Autodesk Inventor part; units mm, degrees
ref_plane "YZ Plane" through (0, 0, 0) normal (1, 0, 0) x (0, 1, 0)
ref_plane "XZ Plane" through (0, 0, 0) normal (0, 1, 0) x (-1, 0, 0)
ref_plane "XY Plane" through (0, 0, 0) normal (0, 0, 1) x (1, 0, 0)
sketch "Sketch1" plane through (0, 0, 0) normal (1, 0, 0) x (0, 1, 0)
  line L0 (0, 0) -> (20, 0)
  line L1 (20, 0) -> (20, -160)
  line L2 (20, -160) -> (0, -160)
  line L3 (0, -160) -> (0, 0)
  line L4 (10, 0) -> (10, -160) construction
  line L5 (20, -6) -> (0, -6) construction
  line L6 (20, -16) -> (0, -16) construction
  line L7 (20, -142.5) -> (0, -142.5) construction
  line L8 (25, -152.5) -> (0, -152.5) construction
  line L9 (20, -89) -> (0, -89) construction
  line L10 (25, -99) -> (0, -99) construction
  point P0 (15, -16)
  point P1 (15, -6)
  point P2 (5, -16)
  point P3 (5, -6)
  point P4 (15, -152.5)
  point P5 (15, -142.5)
  point P6 (5, -142.5)
  point P7 (5, -152.5)
  point P8 (15, -99)
  point P9 (15, -89)
  point P10 (5, -89)
  point P11 (5, -99)
  dimension "d1" = 20
  dimension "d10" = 6
  dimension "d11" = 10
  dimension "d12" = 10
  dimension "d13" = 10
  dimension "d14" = 10
  dimension "d16" = 10
  dimension "d17" = 10
  dimension "d27" = 10
  dimension "d28" = 10
  dimension "d29" = 10
  dimension "d30" = 89
  dimension "d40" = 142.5
  dimension "d41" = 160
extrude "Extrusion1" add sketch "Sketch1" along normal blind 2
hole "Hole1" at (0, 15, -16) at (0, 15, -6) at (0, 5, -16) at (0, 5, -6) at (0, 15, -142.5) at (0, 15, -152.5) at (0, 5, -152.5) at (0, 5, -142.5) at (0, 15, -89) at (0, 15, -99) at (0, 5, -99) at (0, 5, -89) direction (1, 0, 0) diameter 5 end through all
sketch "Sketch2" plane through (2, 0, 0) normal (1, 0, 0) x (0, 0, -1)
  arc A0 (27.5, 16) -> (27.5, 4) centre (27.5, 10) ccw
  line L0 (27.5, 10) -> (27.5, 4) construction
  line L1 (27.5, 10) -> (27.5, 16) construction
  line L2 (0, 20) -> (0, 0)
  line L3 (0, 10) -> (160, 10) construction
  line L4 (160, 0) -> (160, 20)
  line L5 (27.5, 16) -> (77.5, 16)
  line L6 (27.5, 4) -> (77.5, 4)
  circle A1 centre (89, 15) radius 2.5 construction
  circle A2 centre (89, 5) radius 2.5 construction
  line L7 (89, 15) -> (89, 5) construction
  circle A3 centre (16, 15) radius 2.5 construction
  circle A4 centre (16, 5) radius 2.5 construction
  line L8 (16, 15) -> (16, 5) construction
  circle A5 centre (99, 15) radius 2.5 construction
  line L9 (99, 15) -> (89, 15) construction
  line L10 (94, 15) -> (94, -7.3428) construction
  arc A6 (77.5, 4) -> (77.5, 16) centre (77.5, 10) ccw
  line L11 (77.5, 10) -> (77.5, 4) construction
  line L12 (77.5, 10) -> (77.5, 16) construction
  line L13 (110.5, 4) -> (131, 4)
  line L14 (131, 16) -> (110.5, 16)
  arc A7 (110.5, 16) -> (110.5, 4) centre (110.5, 10) ccw
  arc A8 (131, 4) -> (131, 16) centre (131, 10) ccw
  circle A9 centre (99, 5) radius 2.5 construction
  circle A10 centre (16, 15) radius 2.5 construction
  circle A11 centre (142.5, 5) radius 2.5 construction
  dimension "d31" = 180
  dimension "d32" = 6
  dimension "d33" = 50
  dimension "d34" = 73
  dimension "d36" = 180
  dimension "d42" = 6
  dimension "d43" = 6
  dimension "d44" = 20.5
  dimension "d46" = 180
  dimension "d47" = 5
  dimension "d48" = 11.5
  dimension "d49" = 43.5
  dimension "d50" = 11.5
extrude "Extrusion2" cut sketch "Sketch2" against normal blind 10
equation "\"d42\" = d32"
equation "\"d43\" = d32"
equation "\"d46\" = d36"
equation "\"d48\" = 0 * d47 + 0.5 * d34 - 0.5 * d33"
equation "\"d50\" = -0.5 * d44 + 0.5 * d49 + 0 * d47"
properties part number "sideLongitudinal" material "Steel"
Geometry: final body of the model. Coordinates: model frame, mm. A direction names the side the tool comes from. Round coordinates to 2 decimals unless told otherwise and drop trailing zeros. Order: outer loops, then holes, each group sorted by start corner. A loop starts at its lowest first (then second) coordinate and runs counter-clockwise, first axis right, second up. Notation, with made-up numbers: (-29, -39.75) - (-19, -39.75) arc R16 ccw to (-19, -15.75) - close; hole circle Ø1 at (30.25, 6.5). An arc over 180 degrees is marked (long way). Write item = value, one per line. Start each with the question number.
Q1. Access query for faces 3 (the flat face through (2, 3, -79)), 4 (the cylindrical face through (1, 10.1, -21.5)). Directions: +Z, -Z, +X, -X, +Y, -Y. A direction counts if a zero-diameter tool reaches every point of the face in a straight line with its end or side. Return the directions, or none.
Q2. Cut plane D-D on z = -134.5. Return the cut outline in (x, y).
Q3. Cut plane C-C on z = -44.5. Return the cut outline in (x, y), and give its area (3 significant figures).
Q4. Cut plane B-B on z = -99. Return the cut outline in (x, y).
Q5. Pull-direction query (Z, two-part tool) for faces 1 (the flat face through (0, 3, -79)), 2 (the cylindrical face through (1.01, 15.96, -140.19)); classes: +Z half, -Z half, draft (parallel to the pull), parting line (faces both ways), or undercut.
Q6. Ray query, line 1 (Y direction, x = 1.35, z = -152.5); line 2 (Y direction, x = 1.3, z = -152); line 3 (Y direction, x = 1, z = -113). Return the intervals inside material, ascending. Write a range as from..to.
Q7. Cut plane A-A on y = 10. Return the cut outline in (x, z).
Outcome:
q1.face_3 = +Z, -Z, +X, +Y, -Y
q1.face_4 = +X, -X
q2.outline = (0, 0) - (2, 0) - (2, 5.13) - (0, 5.13) - close; (0, 14.87) - (2, 14.87) - (2, 20) - (0, 20) - close
q3.outline = (0, 0) - (2, 0) - (2, 4) - (0, 4) - close; (0, 16) - (2, 16) - (2, 20) - (0, 20) - close
q3.area = 16.0 mm^2
q4.outline = (0, 0) - (2, 0) - (2, 2.5) - (0, 2.5) - close; (0, 7.5) - (2, 7.5) - (2, 12.5) - (0, 12.5) - close; (0, 17.5) - (2, 17.5) - (2, 20) - (0, 20) - close
q5.face_1 = draft
q5.face_2 = undercut
q6.line_1 = 0..2.5, 7.5..12.5, 17.5..20
q6.line_2 = 0..2.55, 7.45..12.55, 17.45..20
q6.line_3 = 0..4, 16..20
q7.outline = (0, -160) - (2, -160) - (2, -137) - (0, -137) - close; (0, -104.5) - (2, -104.5) - (2, -83.5) - (0, -83.5) - close; (0, -21.5) - (2, -21.5) - (2, 0) - (0, 0) - close
